```python
from build123d import *

# Parameters (mm, degrees)
BOSS_EXTRUDE1_DEPTH = 2.5


with BuildPart() as part:
    # Sketch1 → Boss-Extrude1 (new body)
    with BuildSketch(Plane.XY):
        Polygon((-40, -26.705), (-25, -26.705), (-25, -29.205), (-15, -29.205), (-15, -26.705), (-5, -26.705), (-5, -29.205), (5, -29.205), (5, -26.705), (15, -26.705), (15, -29.205), (25, -29.205), (25, -26.705), (35, -26.705), (40, -26.705), (40, 26.705), (-40, 26.705), align=None)
        with BuildLine():
            Line((-27, -17.5), (27, -17.5))
            ThreePointArc((27, -17.5), (29.121320344, -16.621320344), (30, -14.5))
            Line((30, -14.5), (30, 14.5))
            ThreePointArc((30, 14.5), (29.121320344, 16.621320344), (27, 17.5))
            Line((27, 17.5), (-27, 17.5))
            ThreePointArc((-27, 17.5), (-29.121320344, 16.621320344), (-30, 14.5))
            Line((-30, 14.5), (-30, -14.5))
            ThreePointArc((-30, -14.5), (-29.121320344, -16.621320344), (-27, -17.5))
        make_face(mode=Mode.SUBTRACT)
    extrude(amount=BOSS_EXTRUDE1_DEPTH)


solid = part.part
```
The model under review builds one solid part; all positions refer to its coordinate system, in mm. A direction names the side the tool comes from. Give positions to 0.01 mm unless a question says otherwise; leave off trailing zeros. Write each loop counter-clockwise with the first axis right and the second up, starting at its lowest first coordinate (ties: lowest second). Pieces come first, ordered by that corner, then holes. Notation, with made-up numbers: (-28, 76) -> (23, 76) arc R23 cw to (23, 104) -> close; hole circle Ø8 at (-27.5, -12). An arc over 180 degrees is marked (long way). Put each result on its own line as item: value.
(1) We need section B-B, the plane y = 2.5. Give the boundary of the cut face in (x, z).
Results are:
outline: (-40, 0) -> (-30, 0) -> (-30, 2.5) -> (-40, 2.5) -> close; (30, 0) -> (40, 0) -> (40, 2.5) -> (30, 2.5) -> close
(2) We need section C-C, the plane z = 2. Give the boundary of the cut face in (x, y) (3 decimals), and give its area (3 significant figures).
Results are:
outline: (-40, -26.705) -> (-25, -26.705) -> (-25, -29.205) -> (-15, -29.205) -> (-15, -26.705) -> (-5, -26.705) -> (-5, -29.205) -> (5, -29.205) -> (5, -26.705) -> (15, -26.705) -> (15, -29.205) -> (25, -29.205) -> (25, -26.705) -> (40, -26.705) -> (40, 26.705) -> (-40, 26.705) -> close; hole (-30, -14.5) arc R3 ccw to (-27, -17.5) -> (27, -17.5) arc R3 ccw to (30, -14.5) -> (30, 14.5) arc R3 ccw to (27, 17.5) -> (-27, 17.5) arc R3 ccw to (-30, 14.5) -> close
area: 2,260 mm²
(3) We need section A-A, the plane x = 14. Give the boundary of the cut face in (y, z) (3 decimals).
Results are:
outline: (-26.705, 0) -> (-17.5, 0) -> (-17.5, 2.5) -> (-26.705, 2.5) -> close; (17.5, 0) -> (26.705, 0) -> (26.705, 2.5) -> (17.5, 2.5) -> close
(4) To check wall thickness, follow probe 1 along X at (y, z) = (-27, 1.1); probe 2 along X at (y, z) = (-1.5, 0.1); probe 3 along Y at (x, z) = (8.5, 0.8) (3 decimals). State the ranges of each line that lie inside material, in increasing order. Write a range as from..to.
Results are:
probe 1: -25..-15, -5..5, 15..25
probe 2: -40..-30, 30..40
probe 3: -26.705..-17.5, 17.5..26.705
(5) The part is to be moulded in two halves that separate along Y. For faces 1 (the cylindrical face through (29.1, -16.64, 1.23)), 2 (the flat face through (5, -28, 1)), 3 (the flat face through (0, -29.205, 1)), say which applies: pulls with the +Y half, pulls with the -Y half, needs draft (parallel to the pull), parting line crosses it, or undercut.
Results are:
face 1: undercut
face 2: needs draft
face 3: pulls with the -Y half
(6) For pin 1 Ø1.2 at (x, z) = (10, 1.5) entering from -Y (3 decimals); pin 2 Ø0.8 at (y, z) = (-28.5, 1.5) entering from +X; pin 3 Ø1.2 at (y, z) = (-27.5, 1.5) entering from -X, all flat-tipped, find the tip position at first contact; note any pin that passes through.
Results are:
pin 1: y = -26.705
pin 2: x = 25
pin 3: x = -25
(7) Tool access review of faces 4 (the flat face through (32, -26.705, 1)), 5 (the flat face through (-25, -28, 1)), 6 (the cylindrical face through (-29.1, 16.64, 1.23)), 7 (the flat face through (15, -28, 1)): name each direction out of +Z, -Z, +X, -X, +Y, -Y from which nothing blocks a thin tool from reaching the whole face with its end or side.
Results are:
face 4: +Z, -Z, +X, -Y
face 5: +Z, -Z, -X, -Y
face 6: +Z, -Z
face 7: +Z, -Z, -Y
